For this review, take the finished solid that the model builds, in its own axes (mm). A direction names the side the tool comes from. Coordinates: 2 decimals unless noted, no trailing zeros. Loops run counter-clockwise (first coordinate to the right, second up) from the corner with the lowest first, then second, coordinate; pieces in that order, holes last.
1. Take a section at B-B, the plane x = 58.5. State the section outline as (y, z) points, then the cut area to 3 significant figures.
2. To check wall thickness, follow probe 1 along Z at (x, y) = (53, 61.5); probe 2 along X at (y, z) = (12, 28.5); probe 3 along Z at (x, y) = (111, 42). State the ranges of each line that lie inside material, in increasing order.
3. Take a section at A-A, the plane z = 44. State the section outline as (x, y) points, then the cut area to 3 significant figures.
4. Take a section at D-D, the plane z = 8. State the section outline as (x, y) points, then the cut area to 3 significant figures.
5. Take a section at C-C, the plane y = 21. State the section outline as (x, z) points.
6. Mouldability with a two-part tool opening along X and no side actions: class faces 1 (the face through (75, 38, 0)), 2 (the face through (152.4, 38, 23)), 3 (the face through (12.7, 38, 32)) as pulls with the +X half, pulls with the -X half, needs draft (parallel to the pull), parting line crosses it, or undercut.
7. Clearance check with flat-ended pins moving along their axes: P1, Ø7.5, axis at x = 134, y = 33.5, coming from the -Z side; P2, Ø14, axis at y = 23.5, z = 45.5, coming from the -X side; P3, Ø4, axis at y = 50.5, z = 4.5, coming from the +X side; P4, Ø6, axis at x = 133, y = 14.5, coming from the +Z side. State where each tip first meets the part, or that it passes through.
8. Machinability: for faces 4 (the face through (115, 38, 38.1)), 5 (the face through (75, 76.2, 20)), 6 (the face through (50.8, 38, 45)), 7 (the face through (140, 38, 12.7)), 8 (the face through (38, 38, 25.4)), which of the approach directions +Z, -Z, +X, -X, +Y, -Y give a long, thin tool a straight path to every point of the face, cutting with its end or side? Answer none if there is none.
```python
from build123d import *

# Parameters (mm, degrees)
F1_DEPTH = 76.2
F3_DEPTH = 25.4
F5_DEPTH = 76.2


with BuildPart() as f1:
    # F0 (on Front) → F1 (new body)
    with BuildSketch(Plane.XZ):
        Polygon((0, 50.8), (0, 0), (152.4, 0), (152.4, 38.1), (76.2, 38.1), (76.2, 50.8), (50.8, 50.8), (50.8, 38.1), (63.5, 38.157292), (63.5, 25.4), (12.7, 25.4), (12.7, 38.1), (25.4, 38.1), (25.4, 50.8), align=None)
    extrude(amount=-F1_DEPTH)

    # F2 (on face) → F3 (cut)
    with BuildSketch(Plane.YZ.offset(152.4)):
        Polygon((12.7, 12.7), (25.4, 0), (50.8, 0), (63.5, 12.7), align=None)
    extrude(amount=-F3_DEPTH, mode=Mode.SUBTRACT)

    # F4 (on face) → F5 (cut)
    with BuildSketch(Plane.XZ):
        Polygon((76.2, 50.8), (63.5, 50.8), (76.2, 38.1), align=None)
    extrude(amount=-F5_DEPTH, mode=Mode.SUBTRACT)


solid = f1.part
```
Results list:
1. outline: (0, 0) - (76.2, 0) - (76.2, 25.4) - (0, 25.4) - close; (0, 38.13) - (76.2, 38.13) - (76.2, 50.8) - (0, 50.8) - close
1. area: 2,900 mm2
2. probe 1: z = 0 to 25.4, 38.11 to 50.8
2. probe 2: x = 0 to 12.7, 63.5 to 152.4
2. probe 3: z = 0 to 38.1
3. outline: (0, 0) - (25.4, 0) - (25.4, 76.2) - (0, 76.2) - close; (50.8, 0) - (70.3, 0) - (70.3, 76.2) - (50.8, 76.2) - close
3. area: 3,420 mm2
4. outline: (0, 0) - (152.4, 0) - (152.4, 17.4) - (127, 17.4) - (127, 58.8) - (152.4, 58.8) - (152.4, 76.2) - (0, 76.2) - close
4. area: 10,600 mm2
5. outline: (0, 0) - (152.4, 0) - (152.4, 4.4) - (127, 4.4) - (127, 12.7) - (152.4, 12.7) - (152.4, 38.1) - (76.2, 38.1) - (63.5, 50.8) - (50.8, 50.8) - (50.8, 38.1) - (63.5, 38.16) - (63.5, 25.4) - (12.7, 25.4) - (12.7, 38.1) - (25.4, 38.1) - (25.4, 50.8) - (0, 50.8) - close
6. face 1: needs draft
6. face 2: pulls with the +X half
6. face 3: undercut
7. P1: stops at z = 12.7
7. P2: stops at x = 0
7. P3: stops at x = 127
7. P4: stops at z = 38.1
8. face 4: +Z, +X, +Y, -Y
8. face 5: +Z, -Z, +X, -X, +Y
8. face 6: +Z, +Y, -Y
8. face 7: +X
8. face 8: +Y, -Y
